Geometry check sheet. Reference: the model listing, model coordinates, mm. Face numbers are marked on the shaded views. Coordinates: 2 decimals unless noted, no trailing zeros. Write each loop counter-clockwise with the first axis right and the second up, starting at its lowest first coordinate (ties: lowest second). Pieces come first, ordered by that corner, then holes. Notation, with made-up numbers: (-8.5, -23.5) -> (14.5, -23.5) arc R24 cw to (14.5, -3.5) -> close; hole circle Ø5 at (1, 53). An arc over 180 degrees is marked (long way). Use a Markdown table: item, result.
Autodesk Fusion 360 part; units mm, degrees
sketch "Ring" plane through (0, 0, 0) normal (1, 0, 0) x (0, 1, 0)
  line L0 (0, 0) -> (0, 5.5)
  line L1 (0, 0) -> (13.5, 0)
  line L2 (13.5, 0) -> (13.5, 1)
  line L3 (13.5, 1) -> (0.5, 1)
  line L4 (0.5, 1) -> (0.5, 4)
  line L5 (0.5, 4) -> (0.5, 4.5)
  line L6 (0.5, 4.5) -> (0.5, 5.5)
  line L7 (0, 5.5) -> (0.5, 5.5)
  line L8 (100.5, -11) -> (100.5, 21) construction
  point P0 (100.5, 0)
  dimension "d11" = 1
  dimension "d12" = 3
  dimension "d13" = 1
  dimension "d21" = 0.5
  dimension "d47" = 13
  dimension "d48" = 100
  dimension "d55" = 0.5
  dimension "d56" = 0.5
revolve "Revolve Ring" add sketch "Ring" angle 360 about axis through (0, 100.5, -11) along (0, 0, 1)
sketch "Cutout" plane through (0, 0, 1) normal (0, 0, 1) x (-1, 0, 0)
  circle A0 centre (0, -100.5) radius 100
  circle A1 centre (0, -100.5) radius 87
  circle A2 centre (0, -100.5) radius 87
  circle A3 centre (0, -100.5) radius 93
  line L0 (39.1124, -22.7876) -> (47.8845, -20.775)
  line L1 (-38.6062, -22.5349) -> (-47.365, -20.4653)
  line L2 (-38.6062, -178.4651) -> (-47.365, -180.5347)
  line L3 (39.1124, -178.2124) -> (47.8845, -180.225)
  line L4 (47.8845, -180.225) -> (47.8845, -20.775) construction
  line L5 (-47.365, -180.5347) -> (-47.365, -20.4653) construction
  point P0 (39.1124, -22.7876)
  dimension "d24" = 0
  dimension "d25" = 186
  dimension "d37" = 9
  dimension "d49" = 95.25
  dimension "d50" = 77.719
  dimension "d52" = 159.45
extrude "Remove Cutout" cut sketch "Cutout" against normal blind 10 contours A1 A2 A3 L0 L3 | A1 A2 A3 L1 L2
fillet "Fillet2" radius 1 1 edges at (-93.2327, 64.3385, 1)
equation "d11 = bottom_thickness"
equation "d12 = cardboard_thickness"
equation "d21 = edge_thickness"
equation "d25 = spool_diameter - ( 2 * width_to_holes )"
equation "bottom_thickness = 1 mm"
equation "cardboard_thickness = 3 mm"
equation "spool_diameter = 200 mm"
equation "edge_thickness = 0.5 mm"
equation "width_to_holes = 7 mm"
equation "total_width = 13 mm"
equation "d47 = total_width"
equation "d48 = spool_diameter / 2"
equation "d55 = edge_thickness"
equation "fillet_radius = 1 mm"
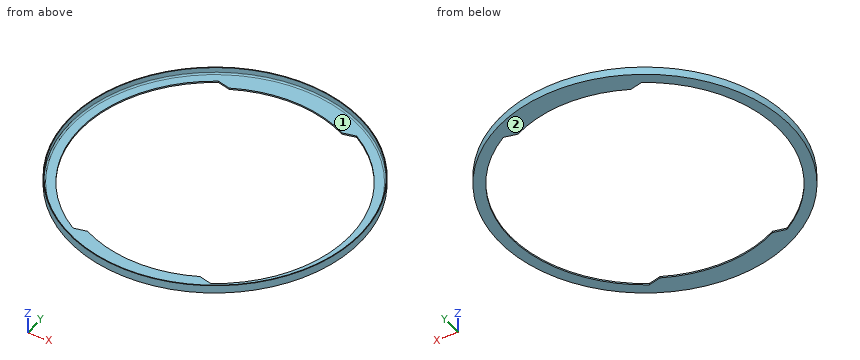
Item 1: Depth check by flat-ended pin: P1, Ø1.5, axis at y = 180, z = 5, coming from the -X side. Enter the tip coordinate at first touch or a pass-through.
Answer block:
| item | result |
|---|---|
| P1 | stops at x = -62.44 |
Item 2: Section check B-B on x = 0. Record the boundary of the cut face in (y, z), then the cut area to 3 significant figures.
Answer block:
| item | result |
|---|---|
| outline | (0, 0) -> (13.5, 0) -> (13.5, 1) -> (1.5, 1) arc R1 cw to (0.5, 2) -> (0.5, 5.5) -> (0, 5.5) -> close; (187.5, 0) -> (201, 0) -> (201, 5.5) -> (200.5, 5.5) -> (200.5, 2) arc R1 cw to (199.5, 1) -> (187.5, 1) -> close |
| area | 31.9 mm^2 |
Item 3: Mould release check, pull along Y, two halves, no side actions. Record for the marked faces 1 and 2: +Y half, -Y half, draft (parallel to the pull), parting line (faces both ways), or undercut.
Answer block:
| item | result |
|---|---|
| face 1 | undercut |
| face 2 | draft |
Item 4: Thickness scan on L1, parallel to X at y = 100.5, z = 3.6; L2, parallel to X at y = 92.5, z = 0.65; L3, parallel to Y at x = -38, z = 1.75. Record the ranges inside material, lowest first. Write a range as [from, to].
Answer block:
| item | result |
|---|---|
| L1 | x = [-100.5, -100], [100, 100.5] |
| L2 | x = [-100.18, -92.66], [92.66, 100.18] |
| L3 | y = [7.46, 8.04], [192.96, 193.54] |
Item 5: Section check A-A on y = 100.5. Record the boundary of the cut face in (x, z), then the cut area to 3 significant figures.
Answer block:
| item | result |
|---|---|
| outline | (-100.5, 0) -> (-93, 0) -> (-93, 1) -> (-99, 1) arc R1 cw to (-100, 2) -> (-100, 5.5) -> (-100.5, 5.5) -> close; (93, 0) -> (100.5, 0) -> (100.5, 5.5) -> (100, 5.5) -> (100, 2) arc R1 cw to (99, 1) -> (93, 1) -> close |
| area | 19.9 mm^2 |
Item 6: Section check C-C on z = 4.5. Record the boundary of the cut face in (x, y).
Answer block:
| item | result |
|---|---|
| outline | circle Ø201 at (0, 100.5); hole circle Ø200 at (0, 100.5) |
